Part model, mm, in its own coordinate system. A direction names the side the tool comes from. Coordinates: 2 decimals unless noted, no trailing zeros. Order: outer loops, then holes, each group sorted by start corner. A loop starts at its lowest first (then second) coordinate and runs counter-clockwise, first axis right, second up. Notation, with made-up numbers: (16, 53) - (45, 53) arc R21 cw to (45, 91) - close; hole circle Ø4 at (30, -40). An arc over 180 degrees is marked (long way). Use a Markdown table: item, result. Add a question column.
1) Drop flat-ended pins along their axis: P1, Ø8, axis at x = -33, z = 19, coming from the +Y side; P2, Ø8, axis at y = 39, z = 60.5, coming from the -X side; P3, Ø3, axis at x = 4, y = 27.5, coming from the +Z side. Give the stop position or say it passes through.
2) Saw through at D-D on y = 37.5. List the corners of the cut face in (x, z).
3) Saw through at A-A on y = 30.75. List the corners of the cut face in (x, z), then the cut area to 3 significant figures.
4) Wall check: L1, parallel to Z at x = 1, y = 26.75; L2, parallel to Z at x = -36, y = 33.25; L3, parallel to Y at x = -0.5, z = 55.5. Give the ranges that are in metal, low to high. Write a range as [from, to].
5) Saw through at B-B on x = -6.5. List the corners of the cut face in (y, z), then the cut area to 3 significant figures.
6) Tool access for faces 1 (the face through (-39.285, 34, 13)), 2 (the face through (-32, 30, 25.4)), 3 (the face through (9, 29, 50.8)): list every direction of +Z, -Z, +X, -X, +Y, -Y with a clear straight run to the whole face (end or side of a thin tool).
7) Saw through at C-C on z = 8. List the corners of the cut face in (x, y), then the cut area to 3 significant figures.
```python
from build123d import *

# Parameters (mm, degrees)
F1_DEPTH = 25.4
F2_DEPTH = 76.2
F3_DEPTH = 50.8


with BuildPart() as f1:
    # F0 (on Top) → F1 (new body)
    with BuildSketch(Plane.XY):
        Polygon((-39.285485, 43.026961), (-39.285485, 24.895199), (-11.943938, 24.895199), align=None)
    extrude(amount=F1_DEPTH)

    # F0 (on Top) → F2 (join)
    with BuildSketch(Plane.XY):
        Polygon((-39.285485, 43.026961), (-11.943938, 24.895199), (17.412249, 41.012321), align=None)
    extrude(amount=F2_DEPTH)

    # F0 (on Top) → F3 (join)
    with BuildSketch(Plane.XY):
        Polygon((17.412249, 41.012321), (-11.943938, 24.895199), (17.412249, 24.895199), align=None)
    extrude(amount=F3_DEPTH)


solid = f1.part
```
Results are:
| question | item | result |
|---|---|---|
| 1 | P1 | y = 42.95 |
| 1 | P2 | x = -39.24 |
| 1 | P3 | z = 50.8 |
| 2 | outline | (-39.29, 0) - (17.41, 0) - (17.41, 50.8) - (11.01, 50.8) - (11.01, 76.2) - (-30.95, 76.2) - (-30.95, 25.4) - (-39.29, 25.4) - close |
| 3 | outline | (-39.29, 0) - (17.41, 0) - (17.41, 50.8) - (-1.28, 50.8) - (-1.28, 76.2) - (-20.77, 76.2) - (-20.77, 25.4) - (-39.29, 25.4) - close |
| 3 | area | 2,910 mm2 |
| 4 | L1 | [0, 50.8] |
| 4 | L2 | [0, 25.4] |
| 4 | L3 | [31.18, 41.65] |
| 5 | outline | (24.9, 0) - (41.86, 0) - (41.86, 76.2) - (27.88, 76.2) - (27.88, 50.8) - (24.9, 50.8) - close |
| 5 | area | 1,220 mm2 |
| 6 | face 1 | +Z, -Z, -X, +Y, -Y |
| 6 | face 2 | +Z, -X, -Y |
| 6 | face 3 | +Z, +X, -Y |
| 7 | outline | (-39.29, 24.9) - (17.41, 24.9) - (17.41, 41.01) - (-39.29, 43.03) - close |
| 7 | area | 971 mm2 |
